Build history of the part. All positions in model axes, mm. Round coordinates to 2 decimals unless told otherwise and drop trailing zeros. Write each loop counter-clockwise with the first axis right and the second up, starting at its lowest first coordinate (ties: lowest second). Pieces come first, ordered by that corner, then holes. Notation, with made-up numbers: (77, -15.5) -> (116, -15.5) arc R23 cw to (116, 1.5) -> close; hole circle Ø7 at (1.25, -12.5). An arc over 180 degrees is marked (long way). Answer in a Markdown table with one row per item.
```python
from build123d import *
from OCP.BRepFilletAPI import BRepFilletAPI_MakeChamfer, BRepFilletAPI_MakeFillet

# Parameters (mm, degrees)
BOSS_EXTRU_1_DEPTH      = 15.5
BOSS_EXTRU_2_START      = -35
BOSS_EXTRU_2_DEPTH      = 30
CHANFREIN1_SIZE         = 3.2
CHANFREIN2_SIZE         = 1.2
CHANFREIN2_SIZE2        = 1.697056275
CONG_1_R1               = 10
CONG_1_R2               = 2.5
ENL_V_MAT_EXTRU_1_REACH = 174.399
ESQUISSE3_R             = 1.6
ESQUISSE4_R             = 2
ENL_V_MAT_EXTRU_2_DEPTH = 13
ESQUISSE9_R             = 2.5
ENL_V_MAT_EXTRU_7_DEPTH = 7
ENL_V_MAT_EXTRU_3_REACH = 174.399
ESQUISSE5_R             = 1.6
ESQUISSE6_R             = 2
ENL_V_MAT_EXTRU_4_DEPTH = 13
ESQUISSE10_R            = 2.5
ENL_V_MAT_EXTRU_8_DEPTH = 7
ESQUISSE7_R             = 1.6
ENL_V_MAT_EXTRU_5_DEPTH = 12
ENL_V_START             = -3
ENL_V_MAT_EXTRU_6_DEPTH = 3


with BuildPart() as part:
    # Esquisse1 → Boss.-Extru.1 (new body)
    with BuildSketch(Plane(origin=(0, 0, 0), x_dir=(1, 0, 0), z_dir=(0, 1, 0))):
        with BuildLine():
            ThreePointArc((0, -42.5), (-23.048861143, -35.707142143), (-38.729833462, -17.5))
            Line((-38.729833462, -17.5), (-165, -17.5))
            Line((-165, -17.5), (-165, -47.5))
            Line((-165, -47.5), (0, -47.5))
            Line((0, -47.5), (0, -42.5))
        make_face()
    extrude(amount=BOSS_EXTRU_1_DEPTH)

    # Esquisse11 → Boss.-Extru.2 (add)
    with BuildSketch(Plane.ZY.offset(165).offset(BOSS_EXTRU_2_START)):
        Polygon((17.5, 0), (14.4, 0), (14.4, 6), (16, 6), (16, 2), (17.5, 2), align=None)
    extrude(amount=-BOSS_EXTRU_2_DEPTH)

    # Chanfrein1
    # the kernel refuses this chamfer: 3.2 mm, written as the material it adds along each edge
    with BuildSketch(Plane(origin=(-100, 10.229385561, 17.5), x_dir=(0.9996219169112968, 0, 0.027495876610586226), z_dir=(0, -1, 0))) as chanfrein1_piece_1_section:
        Polygon((CHANFREIN1_SIZE * 0.999621916911, -CHANFREIN1_SIZE * 0.0274958766106), (-CHANFREIN1_SIZE * 0.0274958766106, -CHANFREIN1_SIZE * 0.999621916911), (0, 0), align=None)
    chanfrein1_piece_1 = extrude(amount=10.229385561, mode=Mode.PRIVATE)
    chanfrein1_piece_1 = split(chanfrein1_piece_1, bisect_by=Plane(origin=(-99.489179746, 2, 15.404286374), z_dir=(0, 1, 0)), keep=Keep.TOP, mode=Mode.PRIVATE)
    chanfrein1_piece_1 = split(chanfrein1_piece_1, bisect_by=Plane(origin=(-99.489179746, 4, 14.4), z_dir=(0, 0, 1)), keep=Keep.TOP, mode=Mode.PRIVATE)
    chanfrein1_piece_1 = split(chanfrein1_piece_1, bisect_by=Plane(origin=(-99.489179746, 6, 15.404286374), z_dir=(0, -1, 0)), keep=Keep.TOP, mode=Mode.PRIVATE)
    chanfrein1_piece_1 = split(chanfrein1_piece_1, bisect_by=Plane(origin=(-99.489179746, 4, 16), z_dir=(0, 0, -1)), keep=Keep.TOP, mode=Mode.PRIVATE)
    add(chanfrein1_piece_1)
    with BuildSketch(Plane(origin=(-100, 2, 17.5), x_dir=(0.9996219169112968, 0, 0.027495876610585147), z_dir=(0, -1, 0))) as chanfrein1_piece_2_section:
        Polygon((CHANFREIN1_SIZE * 0.999621916911, -CHANFREIN1_SIZE * 0.0274958766106), (-CHANFREIN1_SIZE * 0.0274958766106, -CHANFREIN1_SIZE * 0.999621916911), (0, 0), align=None)
    chanfrein1_piece_2 = extrude(amount=2, mode=Mode.PRIVATE)
    chanfrein1_piece_2 = split(chanfrein1_piece_2, bisect_by=Plane(origin=(-98.721329155, 1, 16), z_dir=(0, 0, 1)), keep=Keep.TOP, mode=Mode.PRIVATE)
    add(chanfrein1_piece_2)
    with BuildSketch(Plane(origin=(-100, 2, 17.5), x_dir=(0.9996219169112968, 0, 0.027495876610585147), z_dir=(0, -1, 0))) as chanfrein1_piece_3_section:
        Polygon((CHANFREIN1_SIZE * 0.999621916911, -CHANFREIN1_SIZE * 0.0274958766106), (-CHANFREIN1_SIZE * 0.0274958766106, -CHANFREIN1_SIZE * 0.999621916911), (0, 0), align=None)
    chanfrein1_piece_3 = extrude(amount=2, mode=Mode.PRIVATE)
    chanfrein1_piece_3 = split(chanfrein1_piece_3, bisect_by=Plane(origin=(-99.489179746, 1, 14.4), z_dir=(0, 0, 1)), keep=Keep.TOP, mode=Mode.PRIVATE)
    chanfrein1_piece_3 = split(chanfrein1_piece_3, bisect_by=Plane(origin=(-99.489179746, 1, 16), z_dir=(0, 0, -1)), keep=Keep.TOP, mode=Mode.PRIVATE)
    add(chanfrein1_piece_3)
    with BuildSketch(Plane(origin=(-130, 10.229385561, 17.5), x_dir=(-0.9996219169112966, 0, 0.02749587661058634), z_dir=(0, -1, 0))) as chanfrein1_piece_4_section:
        Polygon((CHANFREIN1_SIZE * 0.999621916911, CHANFREIN1_SIZE * 0.0274958766106), (-CHANFREIN1_SIZE * 0.0274958766106, CHANFREIN1_SIZE * 0.999621916911), (0, 0), align=None)
    chanfrein1_piece_4 = extrude(amount=10.229385561, mode=Mode.PRIVATE)
    chanfrein1_piece_4 = split(chanfrein1_piece_4, bisect_by=Plane(origin=(-130.510820254, 2, 15.404286374), z_dir=(0, 1, 0)), keep=Keep.TOP, mode=Mode.PRIVATE)
    chanfrein1_piece_4 = split(chanfrein1_piece_4, bisect_by=Plane(origin=(-130.510820254, 4, 14.4), z_dir=(0, 0, 1)), keep=Keep.TOP, mode=Mode.PRIVATE)
    chanfrein1_piece_4 = split(chanfrein1_piece_4, bisect_by=Plane(origin=(-130.510820254, 6, 15.404286374), z_dir=(0, -1, 0)), keep=Keep.TOP, mode=Mode.PRIVATE)
    chanfrein1_piece_4 = split(chanfrein1_piece_4, bisect_by=Plane(origin=(-130.510820254, 4, 16), z_dir=(0, 0, -1)), keep=Keep.TOP, mode=Mode.PRIVATE)
    add(chanfrein1_piece_4)
    with BuildSketch(Plane(origin=(-130, 2, 17.5), x_dir=(-0.9996219169112966, 0, 0.027495876610585262), z_dir=(0, -1, 0))) as chanfrein1_piece_5_section:
        Polygon((CHANFREIN1_SIZE * 0.999621916911, CHANFREIN1_SIZE * 0.0274958766106), (-CHANFREIN1_SIZE * 0.0274958766106, CHANFREIN1_SIZE * 0.999621916911), (0, 0), align=None)
    chanfrein1_piece_5 = extrude(amount=2, mode=Mode.PRIVATE)
    chanfrein1_piece_5 = split(chanfrein1_piece_5, bisect_by=Plane(origin=(-131.278670845, 1, 16), z_dir=(0, 0, 1)), keep=Keep.TOP, mode=Mode.PRIVATE)
    add(chanfrein1_piece_5)
    with BuildSketch(Plane(origin=(-130, 2, 17.5), x_dir=(-0.9996219169112966, 0, 0.027495876610585262), z_dir=(0, -1, 0))) as chanfrein1_piece_6_section:
        Polygon((CHANFREIN1_SIZE * 0.999621916911, CHANFREIN1_SIZE * 0.0274958766106), (-CHANFREIN1_SIZE * 0.0274958766106, CHANFREIN1_SIZE * 0.999621916911), (0, 0), align=None)
    chanfrein1_piece_6 = extrude(amount=2, mode=Mode.PRIVATE)
    chanfrein1_piece_6 = split(chanfrein1_piece_6, bisect_by=Plane(origin=(-130.510820254, 1, 14.4), z_dir=(0, 0, 1)), keep=Keep.TOP, mode=Mode.PRIVATE)
    chanfrein1_piece_6 = split(chanfrein1_piece_6, bisect_by=Plane(origin=(-130.510820254, 1, 16), z_dir=(0, 0, -1)), keep=Keep.TOP, mode=Mode.PRIVATE)
    add(chanfrein1_piece_6)

    # Chanfrein2: one chamfer whose edges measure the first distance from different faces: ONE call of the kernel's chamfer builder (chamfer() names one face for all edges)
    chanfrein2_edges_1 = [part.edges().sort_by_distance(p)[0] for p in [
        (-98.3, 4, 16),
    ]]
    chanfrein2_side_1 = [part.faces().sort_by_distance(p)[0] for p in [
        (-98.730952381, 2.523809524, 15.569047619),
    ]]
    chanfrein2_edges_2 = [part.edges().sort_by_distance(p)[0] for p in [
        (-131.7, 4, 16),
    ]]
    chanfrein2_side_2 = [part.faces().sort_by_distance(p)[0] for p in [
        (-131.269047619, 2.523809524, 15.569047619),
    ]]
    chanfrein2 = BRepFilletAPI_MakeChamfer(part.part.solid().wrapped)
    for e in chanfrein2_edges_1:
        chanfrein2.Add(CHANFREIN2_SIZE, CHANFREIN2_SIZE2, e.wrapped, chanfrein2_side_1[0].wrapped)  # the first distance lies on this face
    for e in chanfrein2_edges_2:
        chanfrein2.Add(CHANFREIN2_SIZE, CHANFREIN2_SIZE2, e.wrapped, chanfrein2_side_2[0].wrapped)  # the first distance lies on this face
    add(Compound.cast(chanfrein2.Shape()), mode=Mode.REPLACE)

    # Congé1: one fillet with a radius per group of edges: ONE call of the kernel's fillet builder (fillet() takes one radius for all edges)
    cong_1_edges_1 = [part.edges().sort_by_distance(p)[0] for p in [
        (-165, 7.75, 47.5),
    ]]
    cong_1_edges_2 = [part.edges().sort_by_distance(p)[0] for p in [
        (-165, 7.75, 17.5),
        (-38.729833462, 7.75, 17.5),
    ]]
    cong_1 = BRepFilletAPI_MakeFillet(part.part.solid().wrapped)
    for e in cong_1_edges_1:
        cong_1.Add(CONG_1_R1, e.wrapped)
    for e in cong_1_edges_2:
        cong_1.Add(CONG_1_R2, e.wrapped)
    add(Compound.cast(cong_1.Shape()), mode=Mode.REPLACE)

    # Esquisse3 → Enlèv. mat.-Extru.1 (cut, up to next)
    with BuildSketch(Plane(origin=(0, 15.5, 0), x_dir=(1, 0, 0), z_dir=(0, 1, 0)), mode=Mode.PRIVATE) as enl_v_mat_extru_1_sk1:
        with Locations(Location((-155, -37.5, 0), (0, 0, 270))):
            Circle(ESQUISSE3_R)
    enl_v_mat_extru_1_tool1 = extrude(enl_v_mat_extru_1_sk1.sketch, amount=-ENL_V_MAT_EXTRU_1_REACH, mode=Mode.PRIVATE) & part.part
    # Esquisse3 → Enlèv. mat.-Extru.1 (cut, up to next)
    with BuildSketch(Plane(origin=(0, 15.5, 0), x_dir=(1, 0, 0), z_dir=(0, 1, 0)), mode=Mode.PRIVATE) as enl_v_mat_extru_1_sk2:
        with Locations(Location((-45, -37.5, 0), (0, 0, 270))):
            Circle(ESQUISSE3_R)
    enl_v_mat_extru_1_tool2 = extrude(enl_v_mat_extru_1_sk2.sketch, amount=-ENL_V_MAT_EXTRU_1_REACH, mode=Mode.PRIVATE) & part.part
    add(enl_v_mat_extru_1_tool1.solids().sort_by_distance((-155, 15.5, 37.5))[0], mode=Mode.SUBTRACT)
    add(enl_v_mat_extru_1_tool2.solids().sort_by_distance((-45, 15.5, 37.5))[0], mode=Mode.SUBTRACT)

    # Esquisse4 → Enlèv. mat.-Extru.2 (cut)
    with BuildSketch(Plane.XZ):
        with Locations(Location((-155, 37.5, 0), (0, 0, 270))):
            Circle(ESQUISSE4_R)
        with Locations(Location((-45, 37.5, 0), (0, 0, 270))):
            Circle(ESQUISSE4_R)
    extrude(amount=-ENL_V_MAT_EXTRU_2_DEPTH, mode=Mode.SUBTRACT)

    # Esquisse9 → Enlèv. mat.-Extru.7 (cut)
    with BuildSketch(Plane.XZ):
        with Locations(Location((-155, 37.5, 0), (0, 0, 270))):
            Circle(ESQUISSE9_R)
        with Locations(Location((-45, 37.5, 0), (0, 0, 270))):
            Circle(ESQUISSE9_R)
    extrude(amount=-ENL_V_MAT_EXTRU_7_DEPTH, mode=Mode.SUBTRACT)

    # Esquisse5 → Enlèv. mat.-Extru.3 (cut, up to next)
    with BuildSketch(Plane.XZ, mode=Mode.PRIVATE) as enl_v_mat_extru_3_sk1:
        with Locations(Location((-150, 32.5, 0), (0, 0, 270))):
            Circle(ESQUISSE5_R)
    enl_v_mat_extru_3_tool1 = extrude(enl_v_mat_extru_3_sk1.sketch, amount=-ENL_V_MAT_EXTRU_3_REACH, mode=Mode.PRIVATE) & part.part
    # Esquisse5 → Enlèv. mat.-Extru.3 (cut, up to next)
    with BuildSketch(Plane.XZ, mode=Mode.PRIVATE) as enl_v_mat_extru_3_sk2:
        with Locations(Location((-50, 32.5, 0), (0, 0, 270))):
            Circle(ESQUISSE5_R)
    enl_v_mat_extru_3_tool2 = extrude(enl_v_mat_extru_3_sk2.sketch, amount=-ENL_V_MAT_EXTRU_3_REACH, mode=Mode.PRIVATE) & part.part
    add(enl_v_mat_extru_3_tool1.solids().sort_by_distance((-150, 0, 32.5))[0], mode=Mode.SUBTRACT)
    add(enl_v_mat_extru_3_tool2.solids().sort_by_distance((-50, 0, 32.5))[0], mode=Mode.SUBTRACT)

    # Esquisse6 → Enlèv. mat.-Extru.4 (cut)
    with BuildSketch(Plane(origin=(0, 15.5, 0), x_dir=(1, 0, 0), z_dir=(0, 1, 0))):
        with Locations(Location((-150, -32.5, 0), (0, 0, 270))):
            Circle(ESQUISSE6_R)
        with Locations(Location((-50, -32.5, 0), (0, 0, 270))):
            Circle(ESQUISSE6_R)
    extrude(amount=-ENL_V_MAT_EXTRU_4_DEPTH, mode=Mode.SUBTRACT)

    # Esquisse10 → Enlèv. mat.-Extru.8 (cut)
    with BuildSketch(Plane(origin=(0, 15.5, 0), x_dir=(1, 0, 0), z_dir=(0, 1, 0))):
        with Locations(Location((-50, -32.5, 0), (0, 0, 270))):
            Circle(ESQUISSE10_R)
        with Locations(Location((-150, -32.5, 0), (0, 0, 270))):
            Circle(ESQUISSE10_R)
    extrude(amount=-ENL_V_MAT_EXTRU_8_DEPTH, mode=Mode.SUBTRACT)

    # Esquisse7 → Enlèv. mat.-Extru.5 (cut)
    with BuildSketch(Plane(origin=(0, 0, 17.5), x_dir=(-1, 0, 0), z_dir=(0, 0, -1))):
        with Locations((105, 7)):
            Circle(ESQUISSE7_R)
    extrude(amount=-ENL_V_MAT_EXTRU_5_DEPTH, mode=Mode.SUBTRACT)

    # Esquisse8 → Enlèv. mat.-Extru.6 (cut)
    with BuildSketch(Plane(origin=(0, 0, 17.5), x_dir=(-1, 0, 0), z_dir=(0, 0, -1)).offset(ENL_V_START)):
        Polygon((102.25, 5.41228676), (105, 3.824573519), (107.75, 5.41228676), (107.75, 8.58771324), (102.25, 8.58771324), align=None)
        Polygon((102.25, 8.58771324), (107.75, 8.58771324), (105, 10.175426481), align=None)
        Polygon((105, 10.175426481), (107.75, 8.58771324), (107.75, 15.5), (102.25, 15.5), (102.25, 8.58771324), align=None)
    extrude(amount=-ENL_V_MAT_EXTRU_6_DEPTH, mode=Mode.SUBTRACT)


solid = part.part
```
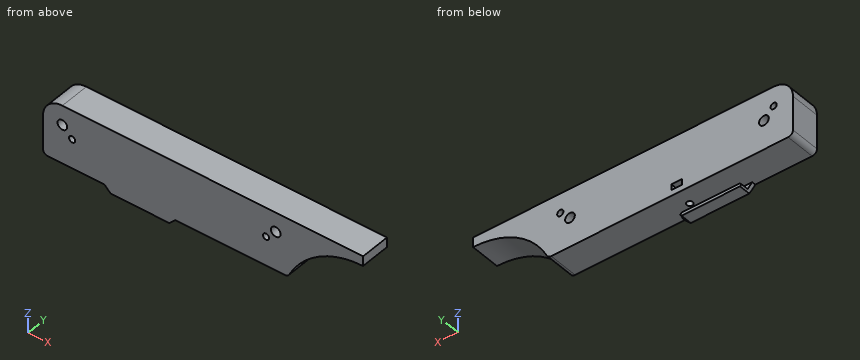
Q1. Saw through at D-D on z = 32.5. Write the cut outline in (x, y), plus the area to 3 significant figures.
A:
| item | result |
|---|---|
| outline | (-165, 0) -> (-151.6, 0) -> (-151.6, 2.5) -> (-152, 2.5) -> (-152, 8.5) -> (-152.5, 8.5) -> (-152.5, 15.5) -> (-165, 15.5) -> close; (-148.4, 0) -> (-51.6, 0) -> (-51.6, 2.5) -> (-52, 2.5) -> (-52, 8.5) -> (-52.5, 8.5) -> (-52.5, 15.5) -> (-147.5, 15.5) -> (-147.5, 8.5) -> (-148, 8.5) -> (-148, 2.5) -> (-148.4, 2.5) -> close; (-48.4, 0) -> (-27.39, 0) -> (-27.39, 15.5) -> (-47.5, 15.5) -> (-47.5, 8.5) -> (-48, 8.5) -> (-48, 2.5) -> (-48.4, 2.5) -> close |
| area | 2,000 mm² |
Q2. Drop flat-ended pins along their axis: P1, Ø3, axis at x = -97, y = 6, coming from the -Z side; P2, Ø0.5, axis at x = -111.5, z = 15, coming from the +Y side. Give the stop position or say it passes through.
A:
| item | result |
|---|---|
| P1 | z = 17.5 |
| P2 | y = 6 |
Q3. Wall check: line 1 (X direction, y = 11.25, z = 34); line 2 (X direction, y = 14.9, z = 37.5); line 3 (Z direction, x = -53, y = 2). Give the ranges that are in metal, low to high. Write a range as [from, to].
A:
| item | result |
|---|---|
| line 1 | [-165, -152], [-148, -52], [-48, -25.5] |
| line 2 | [-165, -156.6], [-153.4, -46.6], [-43.4, -20] |
| line 3 | [17.5, 47.5] |
Q4. Saw through at C-C on x = -126. Write the cut outline in (y, z), plus the area to 3 significant figures.
A:
| item | result |
|---|---|
| outline | (0, 14.4) -> (6, 14.4) -> (6, 16) -> (2, 16) -> (2, 17.5) -> (15.5, 17.5) -> (15.5, 47.5) -> (0, 47.5) -> close |
| area | 478 mm² |
Q5. Saw through at B-B on y = 10. Write the cut outline in (x, z), plus the area to 3 significant figures.
A:
| item | result |
|---|---|
| outline | (-165, 20) arc R2.5 ccw to (-162.5, 17.5) -> (-40.31, 17.5) arc R2.5 ccw to (-38.07, 18.89) arc R42.5 cw to (0, 42.5) -> (0, 47.5) -> (-155, 47.5) arc R10 ccw to (-165, 37.5) -> close; hole circle Ø4 at (-155, 37.5); hole circle Ø5 at (-150, 32.5); hole (-107.75, 20.5) -> (-102.25, 20.5) -> (-102.25, 23.5) -> (-107.75, 23.5) -> close; hole circle Ø5 at (-50, 32.5); hole circle Ø4 at (-45, 37.5) |
| area | 4,150 mm² |
Q6. Saw through at A-A on x = -45. Write the cut outline in (y, z), plus the area to 3 significant figures.
A:
| item | result |
|---|---|
| outline | (0, 17.5) -> (15.5, 17.5) -> (15.5, 35.9) -> (13, 35.9) -> (13, 35.5) -> (7, 35.5) -> (7, 35) -> (0, 35) -> close; (0, 40) -> (7, 40) -> (7, 39.5) -> (13, 39.5) -> (13, 39.1) -> (15.5, 39.1) -> (15.5, 47.5) -> (0, 47.5) -> close |
| area | 398 mm² |
